Verification items for the finished model (mm, model axes). A direction names the side the tool comes from. Give positions to 0.01 mm unless a question says otherwise; leave off trailing zeros. Write each loop counter-clockwise with the first axis right and the second up, starting at its lowest first coordinate (ties: lowest second). Pieces come first, ordered by that corner, then holes. Notation, with made-up numbers: (23, -11.5) -> (30, -11.5) arc R18 cw to (30, 6.5) -> close; hole circle Ø5 at (-24, -8.75). An arc over 180 degrees is marked (long way). Answer as CSV lines item,"result". Start each with the question number.
1) Mould release check, pull along Y, two halves, no side actions. Record for faces 1 (the flat face through (-15, 22.5, 3)), 2 (the flat face through (-15, 0, -155)), 3 (the flat face through (-15, -13, -167)): released by +Y, released by -Y, zero draft, split by the parting line, or undercut.
2) Gauge pin test, flat ends, axial feed: pin 1 Ø13 at (x, z) = (-15.5, -34) entering from -Y; pin 2 Ø0.6 at (x, z) = (-11, -162.5) entering from -Y; pin 3 Ø2.5 at (x, y) = (-14.5, 0.5) entering from -Z. Record the tip position at first contact, or that the pin passes through.
3) Sectioned sample at A-A on z = -33. Record the cut outline in (x, y), and give its area (3 significant figures).
4) Material ranges on L1, parallel to Y at x = -15, z = -228; L2, parallel to X at y = 0, z = -229; L3, parallel to X at y = -17.5, z = 175.5, recorded low to high.
5) Tool access check on faces 4 (the cylindrical face through (-14.51, 3.77, -203.16)), 5 (the flat face through (0, 0, 3)), 6 (the flat face through (-15, -16, 243)). Record the directions out of +Z, -Z, +X, -X, +Y, -Y that give a thin tool (end or side, any length) a straight path to the whole face; none if there is none.
```python
from build123d import *

# Parameters (mm, degrees)
SKETCH1_W           = 500
SKETCH1_H           = 45
BOSS_EXTRUDE1_DEPTH = 30
SKETCH2_W           = 16
SKETCH2_H           = 410
CUT_EXTRUDE1_DEPTH  = 13
SKETCH3_R           = 3.8
CUT_EXTRUDE2_DEPTH  = 95
SKETCH4_R           = 5
CUT_EXTRUDE3_DEPTH  = 12
SKETCH5_W           = 13
SKETCH5_H           = 10
CUT_EXTRUDE4_DEPTH  = 6


with BuildPart() as part:
    # Sketch1 → Boss-Extrude1 (new body)
    with BuildSketch(Plane(origin=(0, 0, 0), x_dir=(0, 0, -1), z_dir=(1, 0, 0))):
        Rectangle(SKETCH1_W, SKETCH1_H)
    extrude(amount=-BOSS_EXTRUDE1_DEPTH)

    # Sketch2 → Cut-Extrude1 (cut)
    with BuildSketch(Plane.XZ.offset(22.5)):
        with Locations((-15, 38)):
            Rectangle(SKETCH2_W, SKETCH2_H)
    extrude(amount=-CUT_EXTRUDE1_DEPTH, mode=Mode.SUBTRACT)

    # Sketch3 → Cut-Extrude2 (cut)
    with BuildSketch(Plane(origin=(0, 0, -250), x_dir=(-1, 0, 0), z_dir=(0, 0, -1))):
        with Locations((15, 0)):
            Circle(SKETCH3_R)
    extrude(amount=-CUT_EXTRUDE2_DEPTH, mode=Mode.SUBTRACT)

    # Sketch4 → Cut-Extrude3 (cut)
    with BuildSketch(Plane.XZ.offset(9.5)):
        with Locations(Location((-15, -162, 0), (0, 0, 270))):
            Circle(SKETCH4_R)
    extrude(amount=-CUT_EXTRUDE3_DEPTH, mode=Mode.SUBTRACT)

    # Sketch5 → Cut-Extrude4 (cut)
    with BuildSketch(Plane.XZ.offset(9.5)):
        with Locations((-15, -162)):
            Rectangle(SKETCH5_W, SKETCH5_H)
    extrude(amount=-CUT_EXTRUDE4_DEPTH, mode=Mode.SUBTRACT)


solid = part.part
```
Ans:
1,face 1,"released by +Y"
1,face 2,"undercut"
1,face 3,"zero draft"
2,pin 1,"stops at y = -9.5"
2,pin 2,"stops at y = 2.5"
2,pin 3,"stops at z = -155"
3,outline,"(-30, -22.5) -> (-23, -22.5) -> (-23, -9.5) -> (-7, -9.5) -> (-7, -22.5) -> (0, -22.5) -> (0, 22.5) -> (-30, 22.5) -> close"
3,area,"1,140 mm²"
4,L1,"y = -22.5 to -3.8, 3.8 to 22.5"
4,L2,"x = -30 to -18.8, -11.2 to 0"
4,L3,"x = -30 to -23, -7 to 0"
5,face 4,"-Z"
5,face 5,"+Z, -Z, +X, +Y, -Y"
5,face 6,"-Y"
